from build123d import *

# Parameters (mm, degrees)
F0_R      = 14.2748
F0_R_2    = 12.827
F1_DEPTH  = 266.7
F3_DEPTH  = 12.7
F4_R      = 14.2748
F4_R_2    = 12.827
F5_DEPTH  = 76.2
F7_R      = 1.524
F8_DEPTH  = 5.08
F10_R     = 1.5875
F11_DEPTH = 5.08
F12_R     = 14.2875
F13_DEPTH = 256.54
F14_R     = 14.2748
F14_R_2   = 12.827
F15_DEPTH = 3.81
F16_R     = 14.2748
F16_R_2   = 10.795
F17_DEPTH = 102.87


with BuildPart() as f1:
    # F0 (on Top) → F1 (new body)
    with BuildSketch(Plane.XY):
        Circle(F0_R)
        Circle(F0_R_2, mode=Mode.SUBTRACT)
    extrude(amount=F1_DEPTH)

    # F2 (on face) → F3 (join)
    with BuildSketch(Plane.XY.offset(266.7)):
        with BuildLine():
            Line((-3.175, 12.4278438999), (-3.175, 13.9172299701))
            ThreePointArc((-3.175, 13.9172299701), (0, -14.2748), (3.175, 13.9172299701))
            Line((3.175, 13.9172299701), (3.175, 12.4278438999))
            ThreePointArc((3.175, 12.4278438999), (0, -12.827), (-3.175, 12.4278438999))
        make_face()
    extrude(amount=F3_DEPTH)

    # F4 (on face) → F5 (join)
    with BuildSketch(Plane.XY.offset(279.4)):
        Circle(F4_R)
        Circle(F4_R_2, mode=Mode.SUBTRACT)
    extrude(amount=F5_DEPTH)

    # F7 (on offset) → F8 (join)
    with BuildSketch(Plane.YZ.offset(12.827)):
        with Locations((0, 12.7)):
            Circle(F7_R)
    extrude(amount=F8_DEPTH)

    # F10 (on offset) → F11 (join)
    with BuildSketch(Plane.YZ.offset(-12.827)):
        with Locations((0, 12.7)):
            Circle(F10_R)
    extrude(amount=-F11_DEPTH)

    # F12 (on face) → F13 (cut)
    with BuildSketch(Plane.XY.offset(355.6)):
        Circle(F12_R)
    extrude(amount=-F13_DEPTH, mode=Mode.SUBTRACT)

    # F14 (on face) → F15 (join)
    with BuildSketch(Plane(origin=(0, 0, 0), x_dir=(1, 0, 0), z_dir=(0, 0, -1))):
        Circle(F14_R)
        Circle(F14_R_2, mode=Mode.SUBTRACT)
    extrude(amount=F15_DEPTH)

    # F16 (on face) → F17 (join)
    with BuildSketch(Plane.XY.offset(99.06)):
        Circle(F16_R)
        Circle(F16_R_2, mode=Mode.SUBTRACT)
    extrude(amount=-F17_DEPTH)


solid = f1.part
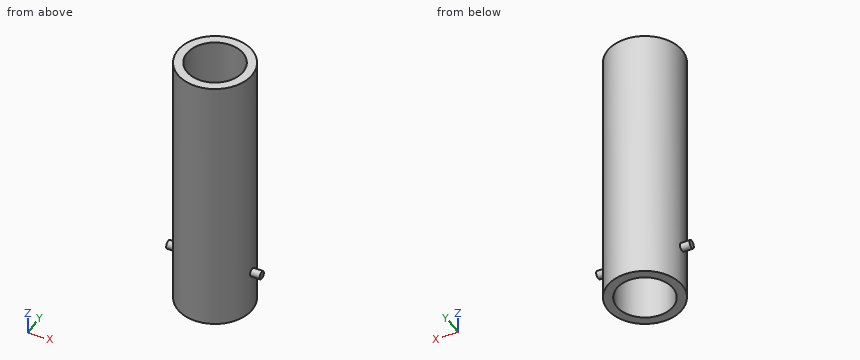
Here's how the part is built. I have some questions about the finished solid (model axes, mm). Coordinates: 2 decimals unless noted, no trailing zeros. Order: outer loops, then holes, each group sorted by start corner. A loop starts at its lowest first (then second) coordinate and runs counter-clockwise, first axis right, second up. Notation, with made-up numbers: (-3.5, -13) - (4.5, -13) arc R22 cw to (4.5, 16) - close; hole circle Ø7 at (-28, -33). An arc over 180 degrees is marked (long way). Use CSV: the item, a comma, the result in double quotes. Start each with the question number.
1. Suppose I cut it at C-C on z = 12.7. List the corners of the cut face in (x, y) for me (1 decimal), then the cut area to 3 significant figures.
2. I'm going to push flat-ended pins straight in: pin 1 (10 mm diameter, centred on x = 12, z = 21, fed in from +Y); pin 2 (5 mm diameter, centred on x = -12, z = 16, fed in from -Y); pin 3 (1.5 mm diameter, centred on x = -7.5, z = 85, fed in from -Y). Where does each tip first touch, or does it pass through?
3. Suppose I cut it at A-A on y = 0. List the corners of the cut face in (x, z) for me (1 decimal).
4. Please list where these lines run through material, in increasing order: line 1 (Y direction, x = 0, z = 33) (3 decimals); line 2 (X direction, y = 0.75, z = 37.5); line 3 (X direction, y = -5.5, z = 9.5). Write a range as from..to.
5. Suppose I cut it at B-B on x = 0. List the corners of the cut face in (y, z) for me (3 decimals), then the cut area to 3 significant figures.
6. Suppose I cut it at D-D on x = 7. List the corners of the cut face in (y, z) for me.
Output:
1,outline,"(-17.9, -1.6) - (-14.2, -1.6) arc R14.3 ccw to (14.2, -1.5) - (17.9, -1.5) - (17.9, 1.5) - (14.2, 1.5) arc R14.3 ccw to (-14.2, 1.6) - (-17.9, 1.6) - close; hole circle Ø21.6 at (0, 0)"
1,area,"297 mm2"
2,pin 1,"stops at y = 12.44"
2,pin 2,"stops at y = -10.65"
2,pin 3,"stops at y = -12.58"
3,outline,"(-17.9, 11.1) - (-14.3, 11.1) - (-14.3, -3.8) - (-10.8, -3.8) - (-10.8, 99.1) - (-14.3, 99.1) - (-14.3, 14.3) - (-17.9, 14.3) - close; (10.8, -3.8) - (14.3, -3.8) - (14.3, 11.2) - (17.9, 11.2) - (17.9, 14.2) - (14.3, 14.2) - (14.3, 99.1) - (10.8, 99.1) - close"
4,line 1,"y = -14.275..-10.795, 10.795..14.275"
4,line 2,"x = -14.26..-10.77, 10.77..14.26"
4,line 3,"x = -13.17..-9.29, 9.29..13.17"
5,outline,"(-14.275, -3.81) - (-10.795, -3.81) - (-10.795, 99.06) - (-14.275, 99.06) - close; (10.795, -3.81) - (14.275, -3.81) - (14.275, 99.06) - (10.795, 99.06) - close"
5,area,"716 mm2"
6,outline,"(-12.44, -3.81) - (-8.22, -3.81) - (-8.22, 99.06) - (-12.44, 99.06) - close; (8.22, -3.81) - (12.44, -3.81) - (12.44, 99.06) - (8.22, 99.06) - close"
